CAD build for the part. Positions are in the model's coordinates, mm. A direction names the side the tool comes from. Round coordinates to 2 decimals unless told otherwise and drop trailing zeros. Write each loop counter-clockwise with the first axis right and the second up, starting at its lowest first coordinate (ties: lowest second). Pieces come first, ordered by that corner, then holes. Notation, with made-up numbers: (-3.75, 40.25) - (48.25, 40.25) arc R21 cw to (48.25, 50.25) - close; hole circle Ø3 at (-36, 12.25). An arc over 180 degrees is marked (long way). Use one line per item in the form item = value. Start each with the question number.
Item 1: Band-saw the part on A-A, the plane z = 16.5. List the corners of the cut face in (x, y).
Item 2: Tool access for faces 5 (the flat face through (0, -8, 50)), 6 (the flat face through (-11, -16, 20)): list every direction of +Z, -Z, +X, -X, +Y, -Y with a clear straight run to the whole face (end or side of a thin tool).
Item 3: Drill centre lines: L1, parallel to Y at x = 0, z = 43; L2, parallel to Z at x = 0, y = -23; L3, parallel to X at y = 3, z = 35. Where is each one in solid material? Low to high.
Item 4: Band-saw the part on D-D, the plane y = 3. Give the number of separate pieces and of enclosed holes in the cut face, and give its area (3 significant figures).
Item 5: Pin check, flat tips, straight feed: pin 1 (6 mm diameter, centred on y = 8, z = 14, fed in from -X); pin 2 (5 mm diameter, centred on x = 3.5, z = 35, fed in from +Y); pin 3 (3 mm diameter, centred on y = -5.5, z = 37, fed in from +X). Stop position of each tip, or through.
Item 6: Band-saw the part on C-C, the plane y = -13. List the corners of the cut face in (x, z), and give its area (3 significant figures).
Item 7: Pull direction Y, two halves, no side cores. Call faces 1 (the cylindrical face through (40, 0, 10)), 2 (the cylindrical face through (-45, 0, 10)), 3 (the cylindrical face through (0, 25, 10)), 4 (the cylindrical face through (1.009, 7.684, 37.325)): +Y half, -Y half, draft (parallel to the pull), parting line (faces both ways), or undercut.
Item 8: Band-saw the part on B-B, the plane x = -33.5. List the corners of the cut face in (y, z).
from build123d import *

# Parameters (mm, degrees)
F1_DEPTH = 20
F3_D     = 10
F3_DEPTH = 20
F3_TIP   = 3.0043030951
F4_R     = 18
F5_DEPTH = 30
F7_D     = 15.5
F7_DEPTH = 25
F7_TIP   = 4.6566697975


# Not quite as in the source:
# - ends of sketch curves that miss each other by under 0.0002 mm in the source are joined


with BuildPart() as f1:
    # F0 (on Top) → F1 (new body)
    with BuildSketch(Plane.XY):
        with BuildLine():
            Line((-10.7142857143, 22.5876975726), (-39.2857142857, 9.0350790291))
            ThreePointArc((-39.2857142857, 9.0350790291), (-45, 0), (-39.2857142857, -9.0350790291))
            Line((-39.2857142857, -9.0350790291), (-10.7742508272, -22.5592536221))
            Line((-10.7742508272, -22.5592536221), (-10.7142857143, -22.5876975726))
            ThreePointArc((-10.7142857143, -22.5876975726), (-0.0331846382, -25.000066073), (10.6543206014, -22.6161415232))
            Line((10.6543206014, -22.6161415232), (39.2857142857, -9.0350790291))
            ThreePointArc((39.2857142857, -9.0350790291), (45, 0), (39.2857142857, 9.0350790291))
            Line((39.2857142857, 9.0350790291), (10.7142857143, 22.5876975726))
            ThreePointArc((10.7142857143, 22.5876975726), (0, 25), (-10.7142857143, 22.5876975726))
        make_face()
    extrude(amount=F1_DEPTH)

    # F3
    with Locations(Plane.XY.offset(20)):
        with Locations((-35, 0), (35, 0)):
            Hole(F3_D / 2, depth=F3_DEPTH)
            with Locations((0, 0, -(F3_DEPTH + F3_TIP / 2))):  # 118° drill point
                Cone(0, F3_D / 2, F3_TIP, mode=Mode.SUBTRACT)

    # F4 (on face) → F5 (join)
    with BuildSketch(Plane.XY.offset(20)):
        Circle(F4_R)
    extrude(amount=F5_DEPTH)

    # F7
    with Locations(Plane.XY.offset(50)):
        with Locations((0, 0)):
            Hole(F7_D / 2, depth=F7_DEPTH)
            with Locations((0, 0, -(F7_DEPTH + F7_TIP / 2))):  # 118° drill point
                Cone(0, F7_D / 2, F7_TIP, mode=Mode.SUBTRACT)


solid = f1.part
Determined:
q1.outline = (-39.29, -9.04) - (-10.71, -22.59) arc R25 ccw to (10.65, -22.62) - (39.29, -9.04) arc R10 ccw to (39.29, 9.04) - (10.71, 22.59) arc R25 ccw to (-10.71, 22.59) - (-39.29, 9.04) arc R10 ccw to start; hole circle Ø10 at (-35, 0); hole circle Ø10 at (35, 0)
q2.face_5 = +Z, +X, -X, +Y, -Y
q2.face_6 = +Z
q3.L1 = -18 to -7.75, 7.75 to 18
q3.L2 = 0 to 20
q3.L3 = -17.75 to -7.15, 7.15 to 17.75
q4.separate_pieces = 3
q4.enclosed_holes = 0
q4.area = 2,140 mm²
q5.pin_1 = -43.66
q5.pin_2 = 17.97
q5.pin_3 = 17.55
q6.outline = (-30.93, 0) - (30.93, 0) - (30.93, 20) - (12.45, 20) - (12.45, 50) - (-12.45, 50) - (-12.45, 20) - (-30.93, 20) - close
q6.area = 1,980 mm²
q7.face_1 = undercut
q7.face_2 = parting line
q7.face_3 = +Y half
q7.face_4 = undercut
q8.outline = (-11.78, 0) - (-4.77, 0) - (-4.77, 20) - (-11.78, 20) - close; (4.77, 0) - (11.78, 0) - (11.78, 20) - (4.77, 20) - close
